Geometry: see drawing. Coordinates: mm, zero at the bounding-box minimum. Round coordinates to 2 decimals unless told otherwise and drop trailing zeros. Loops run counter-clockwise (first coordinate to the right, second up) from the corner with the lowest first, then second, coordinate; pieces in that order, holes last.
(1) Cut plane A-A, the plane z = 60. Output: boundary loops of the cut face in (x, y), and give its area (3 significant figures).
(2) Cut plane D-D, the plane y = 1.5. Give the number of separate pieces and of enclosed holes in the cut face, and give its area (3 significant figures).
(3) Cut plane C-C, the plane z = 110. Output: boundary loops of the cut face in (x, y), and give its area (3 significant figures).
(4) First-contact query: pin 1 Ø6 at (x, z) = (100, 85) entering from +Y. Flat tip, straight axial feed; report the tip coordinate or a pass-through.
(5) Cut plane B-B, the plane x = 49.5. Output: boundary loops of the cut face in (y, z), and give its area (3 significant figures).
(6) Line query: line 1 (X direction, y = 6.65, z = 60); line 2 (X direction, y = 6.65, z = 10); line 3 (X direction, y = 3.05, z = 85). Output: solid intervals per line, ascending.
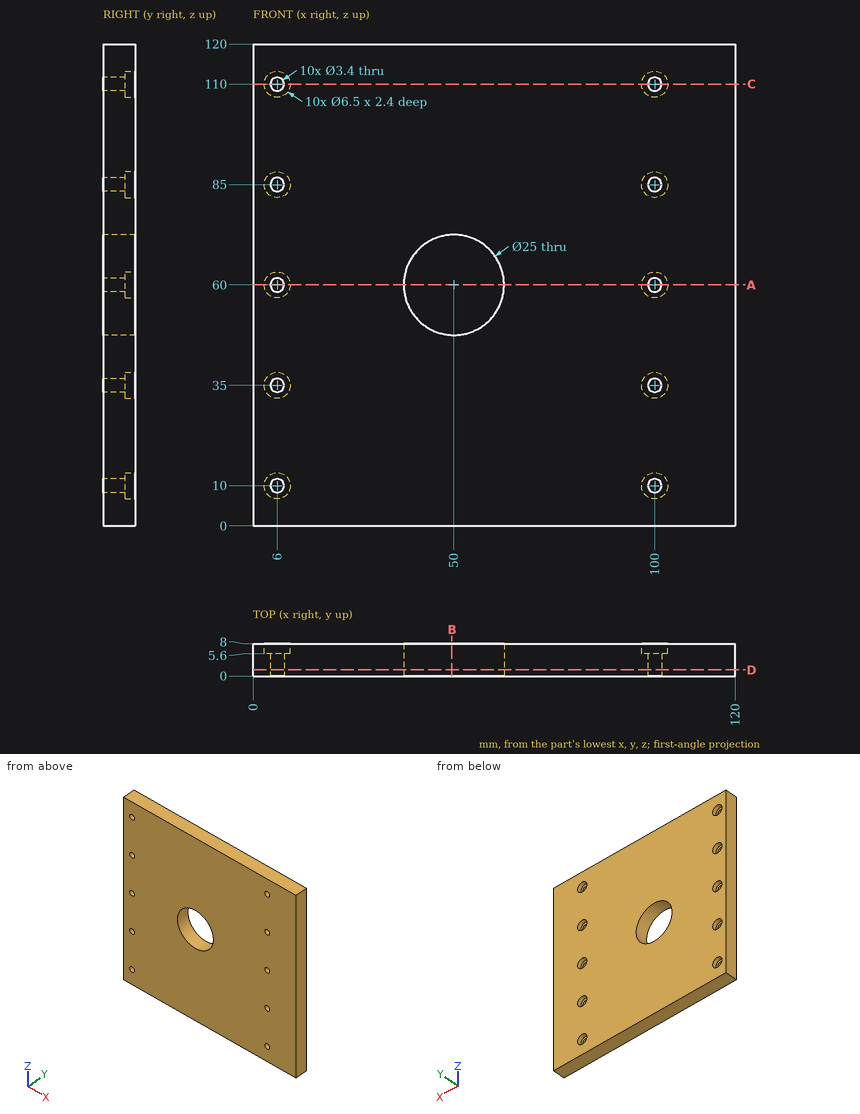
Reported:
1. outline: (0, 0) - (4.3, 0) - (4.3, 5.6) - (2.75, 5.6) - (2.75, 8) - (0, 8) - close; (7.7, 0) - (37.5, 0) - (37.5, 8) - (9.25, 8) - (9.25, 5.6) - (7.7, 5.6) - close; (62.5, 0) - (98.3, 0) - (98.3, 5.6) - (96.75, 5.6) - (96.75, 8) - (62.5, 8) - close; (101.7, 0) - (120, 0) - (120, 8) - (103.25, 8) - (103.25, 5.6) - (101.7, 5.6) - close
1. area: 691 mm2
2. separate pieces: 1
2. enclosed holes: 11
2. area: 13,800 mm2
3. outline: (0, 0) - (4.3, 0) - (4.3, 5.6) - (2.75, 5.6) - (2.75, 8) - (0, 8) - close; (7.7, 0) - (98.3, 0) - (98.3, 5.6) - (96.75, 5.6) - (96.75, 8) - (9.25, 8) - (9.25, 5.6) - (7.7, 5.6) - close; (101.7, 0) - (120, 0) - (120, 8) - (103.25, 8) - (103.25, 5.6) - (101.7, 5.6) - close
3. area: 891 mm2
4. pin 1: stops at y = 5.6
5. outline: (0, 0) - (8, 0) - (8, 47.51) - (0, 47.51) - close; (0, 72.49) - (8, 72.49) - (8, 120) - (0, 120) - close
5. area: 760 mm2
6. line 1: x = 0 to 2.75, 9.25 to 37.5, 62.5 to 96.75, 103.25 to 120
6. line 2: x = 0 to 2.75, 9.25 to 96.75, 103.25 to 120
6. line 3: x = 0 to 4.3, 7.7 to 98.3, 101.7 to 120
